from build123d import *

# Parameters (mm, degrees)
F0_R         = 13.5
F1_DEPTH     = 115
F2_W         = 20.9761769634
F2_H         = 17
F3_DEPTH     = 20
F4_R         = 5
F5_DEPTH     = 25
F6_R         = 10
F7_T4_DEPTH  = 20.9761769634
F7_S5_R      = 5
F7_T6_DEPTH  = 13
F7_S7_R      = 13.5
F7_T8_DEPTH  = 13
F7_T12_DEPTH = 20.9761769634
F7_S13_R     = 13.5
F7_T14_DEPTH = 13
F7_S15_R     = 5
F7_T16_DEPTH = 13
F8_T4_DEPTH  = 42
F8_S5_R      = 13.5
F8_T6_DEPTH  = 23
F8_T10_DEPTH = 42
F8_S11_R     = 13.5
F8_T12_DEPTH = 23


# Not quite as in the source:
# - a fillet or chamfer that OpenCascade refuses, or shapes differently, is made with other operations: its cross-section is extruded or revolved along the edge and cut away or added


with BuildPart() as f1:
    # F0 (on Top) → F1 (new body)
    with BuildSketch(Plane.XY):
        Circle(F0_R)
    extrude(amount=F1_DEPTH)

    # F2 (on face) → F3 (join)
    with BuildSketch(Plane.XY.offset(115)):
        Rectangle(F2_W, F2_H)
    extrude(amount=F3_DEPTH)

    # F4 (on face) → F5 (cut)
    with BuildSketch(Plane.XZ.offset(8.5)):
        with Locations((0, 124.938569963)):
            Circle(F4_R)
    extrude(amount=-F5_DEPTH, mode=Mode.SUBTRACT)

    # F6
    f6_edges = [f1.edges().sort_by_distance(p)[0] for p in [
        (10.488088, 0, 135),
        (-10.488088, 0, 135),
    ]]
    fillet(f6_edges, radius=F6_R)

    # F7: fillet of radius 5 on 2 edges, made by hand


with BuildPart() as f7_tool2:
    # F7_s3 → F7_t4 (new body)
    with BuildSketch(Plane.YZ.offset(-10.4880884817)):
        with BuildLine():
            ThreePointArc((-8.5, 120), (-9.9644660941, 116.4644660941), (-13.5, 115))
            Line((-13.5, 115), (-8.5, 115))
            Line((-8.5, 115), (-8.5, 120))
        make_face()
    extrude(amount=F7_T4_DEPTH)

    # F7_s5 → F7_t6 (cut, symmetric)
    with BuildSketch(Plane.XZ.offset(11)):
        with Locations((0, 124.938569963)):
            Circle(F7_S5_R)
    extrude(amount=F7_T6_DEPTH, both=True, mode=Mode.SUBTRACT)

    # F7_s7 → F7_t8 (intersect, symmetric)
    with BuildSketch(Plane.XY.offset(117.5)):
        Circle(F7_S7_R)
    extrude(amount=F7_T8_DEPTH, both=True, mode=Mode.INTERSECT)


with BuildPart() as f1_1:
    add(f1.part)

    # F7_t1: union F7_tool2
    add(f7_tool2.part)


with BuildPart() as f7_tool10:
    # F7_s11 → F7_t12 (new body)
    with BuildSketch(Plane.YZ.offset(10.4880884817)):
        with BuildLine():
            ThreePointArc((8.5, 120), (9.9644660941, 116.4644660941), (13.5, 115))
            Line((13.5, 115), (8.5, 115))
            Line((8.5, 115), (8.5, 120))
        make_face()
    extrude(amount=-F7_T12_DEPTH)

    # F7_s13 → F7_t14 (intersect, symmetric)
    with BuildSketch(Plane.XY.offset(117.5)):
        Circle(F7_S13_R)
    extrude(amount=F7_T14_DEPTH, both=True, mode=Mode.INTERSECT)

    # F7_s15 → F7_t16 (cut, symmetric)
    with BuildSketch(Plane.XZ.offset(-11)):
        with Locations((0, 124.938569963)):
            Circle(F7_S15_R)
    extrude(amount=F7_T16_DEPTH, both=True, mode=Mode.SUBTRACT)


with BuildPart() as f1_2:
    add(f1_1.part)

    # F7_t9: union F7_tool10
    add(f7_tool10.part)

    # F8: fillet of radius 5 on 2 edges, made by hand


with BuildPart() as f8_tool2:
    # F8_s3 → F8_t4 (new body)
    with BuildSketch(Plane.XZ.offset(21)):
        with BuildLine():
            ThreePointArc((10.4880884817, 120), (11.9525545758, 116.4644660941), (15.4880884817, 115))
            Line((15.4880884817, 115), (10.4880884817, 115))
            Line((10.4880884817, 115), (10.4880884817, 120))
        make_face()
    extrude(amount=-F8_T4_DEPTH)

    # F8_s5 → F8_t6 (intersect, symmetric)
    with BuildSketch(Plane.XY.offset(117.5)):
        Circle(F8_S5_R)
    extrude(amount=F8_T6_DEPTH, both=True, mode=Mode.INTERSECT)


with BuildPart() as f1_3:
    add(f1_2.part)

    # F8_t1: union F8_tool2
    add(f8_tool2.part)


with BuildPart() as f8_tool8:
    # F8_s9 → F8_t10 (new body)
    with BuildSketch(Plane.XZ.offset(-21)):
        with BuildLine():
            ThreePointArc((-15.4880884817, 115), (-11.9525545758, 116.4644660941), (-10.4880884817, 120))
            Line((-10.4880884817, 120), (-10.4880884817, 115))
            Line((-10.4880884817, 115), (-15.4880884817, 115))
        make_face()
    extrude(amount=F8_T10_DEPTH)

    # F8_s11 → F8_t12 (intersect, symmetric)
    with BuildSketch(Plane.XY.offset(117.5)):
        Circle(F8_S11_R)
    extrude(amount=F8_T12_DEPTH, both=True, mode=Mode.INTERSECT)


with BuildPart() as f1_4:
    add(f1_3.part)

    # F8_t7: union F8_tool8
    add(f8_tool8.part)


solid = f1_4.part
Build history of the part. All positions in model axes, mm. A direction names the side the tool comes from. Coordinates: 2 decimals unless noted, no trailing zeros. Write each loop counter-clockwise with the first axis right and the second up, starting at its lowest first coordinate (ties: lowest second). Pieces come first, ordered by that corner, then holes.
(1) Pin check, flat tips, straight feed: pin 1 Ø4.5 at (x, z) = (-2, 127.5) entering from +Y; pin 2 Ø1.5 at (x, z) = (10, 27.5) entering from +Y; pin 3 Ø5 at (x, z) = (7, 99.5) entering from -Y. Stop position of each tip, or through.
(2) 3-axis set-ups, long thin cutter, end or side, ignore diameter. For faces 1 (the flat face through (-10.488, 0, 122)), 2 (the flat face through (0, 8.5, 131)), 3 (the flat face through (10.488, 0, 122)): which of +Z, -Z, +X, -X, +Y, -Y reach the whole face in a straight line?
(3) Mould opens along Z. For faces 4 (the cylindrical face through (-1.084, -0.119, 120.057)), 5 (the cylindrical face through (0.15, 9.37, 117.18)), 6 (the flat face through (0, -8.5, 131)) say: pulls with the +Z half, pulls with the -Z half, needs draft (parallel to the pull), parting line crosses it, or undercut.
(4) Cut at B-B on z = 81.5. List the corners of the cut face in (x, y).
(5) Cut at A-A on y = 0. List the corners of the cut face in (x, z).
(6) Drill centre lines: line 1 (Y direction, x = -5, z = 120.5); line 2 (X direction, y = 0.5, z = 94); line 3 (Z direction, x = 8.25, y = 4.5). Where is each one in solid material? Low to high.
(7) Cut at D-D on y = 7.25. List the corners of the cut face in (x, z), and give its area (3 significant figures).
(8) Cut at C-C on x = 6.75. List the corners of the cut face in (y, z), and give its area (3 significant figures).
Working result:
1. pin 1: stops at y = 8.5
1. pin 2: stops at y = 9.83
1. pin 3: stops at y = -12.73
2. face 1: +Z, -X, +Y, -Y
2. face 2: +Z, +X, -X, +Y
2. face 3: +Z, +X, +Y, -Y
3. face 4: undercut
3. face 5: pulls with the +Z half
3. face 6: needs draft
4. outline: circle Ø27 at (0, 0)
5. outline: (-13.5, 0) - (13.5, 0) - (13.5, 115.41) arc R5 cw to (10.49, 120) - (10.49, 125) arc R10 ccw to (0.49, 135) - (-0.49, 135) arc R10 ccw to (-10.49, 125) - (-10.49, 120) arc R5 cw to (-13.5, 115.41) - close; hole circle Ø10 at (0, 124.94)
6. line 1: y = -8.5 to 8.5
6. line 2: x = -13.49 to 13.49
6. line 3: z = 0 to 131.3
7. outline: (-11.39, 0) - (11.39, 0) - (11.39, 117.14) arc R5 cw to (10.49, 120) - (10.49, 125) arc R10 ccw to (0.49, 135) - (-0.49, 135) arc R10 ccw to (-10.49, 125) - (-10.49, 120) arc R5 cw to (-11.39, 117.14) - close; hole circle Ø10 at (0, 124.94)
7. area: 2,920 mm2
8. outline: (-11.69, 0) - (11.69, 0) - (11.69, 115.34) arc R5 cw to (8.5, 120) - (8.5, 132.8) - (-8.5, 132.8) - (-8.5, 120) arc R5 cw to (-11.69, 115.34) - close
8. area: 3,000 mm2
